from build123d import *

# Parameters (mm, degrees)
F0_W     = 965.2
F0_H     = 2133.6
F0_W_2   = 292.1
F0_H_2   = 647.7
F0_H_3   = 254
F1_DEPTH = 19.05


with BuildPart() as f1:
    # F0 (on Front) → F1 (new body)
    with BuildSketch(Plane.XZ):
        Rectangle(F0_W, F0_H)
        with Locations((-209.55, -615.95)):
            Rectangle(F0_W_2, F0_H_2, mode=Mode.SUBTRACT)
        with Locations((209.55, -615.95)):
            Rectangle(F0_W_2, F0_H_2, mode=Mode.SUBTRACT)
        with Locations((-209.55, 234.95)):
            Rectangle(F0_W_2, F0_H_2, mode=Mode.SUBTRACT)
        with Locations((-209.55, 812.8)):
            Rectangle(F0_W_2, F0_H_3, mode=Mode.SUBTRACT)
        with Locations((209.55, 234.95)):
            Rectangle(F0_W_2, F0_H_2, mode=Mode.SUBTRACT)
        with Locations((209.55, 812.8)):
            Rectangle(F0_W_2, F0_H_3, mode=Mode.SUBTRACT)
    extrude(amount=F1_DEPTH)


solid = f1.part
Input: part model. Units: mm. Frame: model coordinates. Give positions to 0.01 mm unless a question says otherwise; leave off trailing zeros. Write each loop counter-clockwise with the first axis right and the second up, starting at its lowest first coordinate (ties: lowest second). Pieces come first, ordered by that corner, then holes. Notation, with made-up numbers: M -19,75 L 24,75 A23 cw 24,89 Z; hole C 85.25,10 d6. An arc over 180 degrees is marked long. Write item = value, one per line. Start each with the question number.
1) Cut plane C-C on x = 270.5. Return the cut outline in (y, z).
2) Cut plane A-A on z = -891.5. Return the cut outline in (x, y), then the cut area to 3 significant figures.
3) Material intervals for line 1 along X through (y, z) = (-8.25, -462.5); line 2 along Z through (x, y) = (-346.5, -16.5), sorted ascending. Write a range as [from, to].
4) Cut plane B-B on y = -12.25. Return the cut outline in (x, z), then the cut area to 3 significant figures.
Solved:
q1.outline = M -19.05,-1066.8 L 0,-1066.8 L 0,-939.8 L -19.05,-939.8 Z; M -19.05,-292.1 L 0,-292.1 L 0,-88.9 L -19.05,-88.9 Z; M -19.05,558.8 L 0,558.8 L 0,685.8 L -19.05,685.8 Z; M -19.05,939.8 L 0,939.8 L 0,1066.8 L -19.05,1066.8 Z
q2.outline = M -482.6,-19.05 L -355.6,-19.05 L -355.6,0 L -482.6,0 Z; M -63.5,-19.05 L 63.5,-19.05 L 63.5,0 L -63.5,0 Z; M 355.6,-19.05 L 482.6,-19.05 L 482.6,0 L 355.6,0 Z
q2.area = 7,260 mm2
q3.line_1 = [-482.6, -355.6], [-63.5, 63.5], [355.6, 482.6]
q3.line_2 = [-1066.8, -939.8], [-292.1, -88.9], [558.8, 685.8], [939.8, 1066.8]
q4.outline = M -482.6,-1066.8 L 482.6,-1066.8 L 482.6,1066.8 L -482.6,1066.8 Z; hole M -355.6,-939.8 L -63.5,-939.8 L -63.5,-292.1 L -355.6,-292.1 Z; hole M -355.6,-88.9 L -63.5,-88.9 L -63.5,558.8 L -355.6,558.8 Z; hole M -355.6,685.8 L -63.5,685.8 L -63.5,939.8 L -355.6,939.8 Z; hole M 63.5,-939.8 L 355.6,-939.8 L 355.6,-292.1 L 63.5,-292.1 Z; hole M 63.5,-88.9 L 355.6,-88.9 L 355.6,558.8 L 63.5,558.8 Z; hole M 63.5,685.8 L 355.6,685.8 L 355.6,939.8 L 63.5,939.8 Z
q4.area = 1,150,000 mm2
